Here's how the part is built. I have some questions about the finished solid (model axes, mm). Coordinates: 2 decimals unless noted, no trailing zeros. Order: outer loops, then holes, each group sorted by start corner. A loop starts at its lowest first (then second) coordinate and runs counter-clockwise, first axis right, second up. Notation, with made-up numbers: (53, -33.5) - (95, -33.5) arc R34 cw to (95, -3.5) - close; hole circle Ø4 at (4.5, -2). An arc over 180 degrees is marked (long way). Answer as CSV lines item,"result". Start each with the question number.
Q1. Suppose I cut it at B-B (x = -20). Please give me the cut outline in (y, z).
Q2. Thinking about a two-plate mould opening in Y: for faces 1 (the face through (-0.327, 17.894, 0.11)), 2 (the face through (0.355, 10, 0)), 3 (the face through (-1, 1.976, 0)), which applies, released by +Y, released by -Y, zero draft, split by the parting line, or undercut?
Q3. I need wall thicknesses on line 1 (X direction, y = 14.25, z = 3); line 2 (X direction, y = 17, z = -0.25); line 3 (Y direction, x = -7.25, z = 5). Which ranges of each line are inside material? Lowest first, please.
Q4. For pin 1 Ø12 at (x, y) = (-11, 6) entering from +Z; pin 2 Ø6 at (y, z) = (0, -1.5) entering from -X; pin 3 Ø0.9 at (x, z) = (-0.5, 1) entering from -Y, each with a flat end and sliding along its axis, tell me the tip position at first contact or that it passes through.
Q5. Suppose I cut it at A-A (y = 10). Please give me the cut outline in (x, z).
from build123d import *

# Parameters (mm, degrees)
SALIENTE_EXTRUIR1_DEPTH             = 7.21
SALIENTE_EXTRUIR2_DEPTH             = 7.21
SALIENTE_EXTRUIR2_DEPTH_BACK        = 7.21
CORTAR_EXTRUIR2_DEPTH               = 28.232395202
CORTAR_EXTRUIR2_DEPTH_BACK          = 28.232395202
SALIENTE_EXTRUIR3_REACH             = 29.232
SALIENTE_EXTRUIR3_DIRECTION_2_REACH = 29.232


with BuildPart() as part:
    # Croquis1 → Saliente-Extruir1 (new, symmetric)
    with BuildSketch(Plane.XY):
        with BuildLine():
            add(Edge.make_bspline(
                [(-18.945192114, 7.540918896), (-10.215008384, -3.697644103), (-2.846604825, -5.059081104)],
                knots=[0.497667241, 0.497667241, 0.497667241, 0.49955428, 0.49955428, 0.49955428], degree=2, weights=[1, 1, 1]))
            add(Edge.make_bspline(
                [(-2.846604825, -5.059081104), (-0.742366882, -3.9352066), (0.355125, -2.723253227)],
                knots=[0.498812075, 0.498812075, 0.498812075, 0.499412845, 0.499412845, 0.499412845], degree=2, weights=[1, 1, 1]))
            Line((0.355125, -2.723253227), (0.355125, -2.284841781))
            Line((0.355125, -2.284841781), (-1.394875, -2.223730435))
            add(Edge.make_bspline(
                [(-1.394875, -2.223730435), (-0.90753067, -0.123730435), (-1.394875, 1.976269565)],
                knots=[0, 0, 0, 1, 1, 1], degree=2, weights=[1, 3.231801219, 1]))
            Line((-1.394875, 1.976269565), (0.355125, 2.284841781))
            Line((0.355125, 2.284841781), (0.355125, 3.001549529))
            add(Edge.make_bspline(
                [(0.355125, 3.001549529), (-1.44872627, 6.058427314), (-6.994875026, 10.477389992)],
                knots=[0.500820705, 0.500820705, 0.500820705, 0.502013312, 0.502013312, 0.502013312], degree=2, weights=[1, 1, 1]))
            Line((-6.994875026, 10.477389992), (-8.981845695, 12.608155172))
            Line((-8.981845695, 12.608155172), (-23.035921146, 11.871612288))
            Line((-23.035921146, 11.871612288), (-23.035921146, 11.54013782))
            ThreePointArc((-23.035921146, 11.54013782), (-20.949684518, 9.582335705), (-18.945192114, 7.540918896))
        make_face()
    extrude(amount=SALIENTE_EXTRUIR1_DEPTH, both=True)

    # Croquis4 → Saliente-Extruir2 (add, two sides: drawn at the far end of the back side and taken through both)
    with BuildSketch(Plane.XY.offset(-SALIENTE_EXTRUIR2_DEPTH_BACK)):
        Polygon((-1.394875, 1.976269565), (0.355125, 2.284841781), (0.355125, 1.976269565), align=None)
    extrude(amount=SALIENTE_EXTRUIR2_DEPTH + SALIENTE_EXTRUIR2_DEPTH_BACK)

    # Croquis6 → Cortar-Extruir2 (cut, two sides: drawn at the far end of the back side and taken through both)
    with BuildSketch(Plane(origin=(0, 0, 0), x_dir=(0, 0, -1), z_dir=(1, 0, 0)).offset(-CORTAR_EXTRUIR2_DEPTH_BACK)):
        Polygon((7.21, 12.608155172), (7.21, -5.059081104), (5.21, -5.059081104), align=None)
        Polygon((-7.21, 12.608155172), (-7.21, -5.059081104), (-5.21, -5.059081104), align=None)
    extrude(amount=CORTAR_EXTRUIR2_DEPTH + CORTAR_EXTRUIR2_DEPTH_BACK, mode=Mode.SUBTRACT)

    # Saliente-Extruir3: up to this plane
    saliente_extruir3_end = Plane(origin=(-23.035921146, 12.608155172, 7.21), z_dir=(0, 0.1124854344122626, -0.9936533736897816))
    # Croquis8 → Saliente-Extruir3 (add, up to the surface)
    with BuildSketch(Plane.XY, mode=Mode.PRIVATE) as saliente_extruir3_sk1:
        with BuildLine():
            Line((0.355125, 3.001549529), (0.355125, 17.773466106))
            Line((0.355125, 17.773466106), (-1.028564504, 18.017447899))
            Line((-1.028564504, 18.017447899), (-2.428253067, 18.139904781))
            Line((-2.428253067, 18.139904781), (-3.764520897, 17.705725043))
            Line((-3.764520897, 17.705725043), (-5.005093297, 17.046100998))
            Line((-5.005093297, 17.046100998), (-6.1122761, 16.181074987))
            Line((-6.1122761, 16.181074987), (-7.052428119, 15.136930389))
            Line((-7.052428119, 15.136930389), (-7.796983309, 13.945393009))
            Line((-7.796983309, 13.945393009), (-8.323318739, 12.642667108))
            Line((-8.323318739, 12.642667108), (-9.726428332, 12.56913325))
            add(Edge.make_bspline(
                [(-9.726428332, 12.56913325), (-1.861127424, 6.757298639), (0.355125, 3.001549529)],
                knots=[0.500548048, 0.500548048, 0.500548048, 0.502013312, 0.502013312, 0.502013312], degree=2, weights=[1, 1, 1]))
        make_face()
    saliente_extruir3_tool1 = split(extrude(saliente_extruir3_sk1.sketch, amount=SALIENTE_EXTRUIR3_REACH, mode=Mode.PRIVATE), bisect_by=saliente_extruir3_end, keep=Keep.BOTH, mode=Mode.PRIVATE)
    add(saliente_extruir3_tool1.solids().sort_by_distance((-3.047394, 12.114755, 0))[0])

    # Saliente-Extruir3 direction 2: up to this plane
    saliente_extruir3_direction_2_end = Plane(origin=(-23.035921146, 12.608155172, -7.21), z_dir=(0, 0.1124854344122626, 0.9936533736897816))
    # Croquis8 → Saliente-Extruir3 direction 2 (add, up to the surface)
    with BuildSketch(Plane.XY, mode=Mode.PRIVATE) as saliente_extruir3_direction_2_sk1:
        with BuildLine():
            Line((0.355125, 3.001549529), (0.355125, 17.773466106))
            Line((0.355125, 17.773466106), (-1.028564504, 18.017447899))
            Line((-1.028564504, 18.017447899), (-2.428253067, 18.139904781))
            Line((-2.428253067, 18.139904781), (-3.764520897, 17.705725043))
            Line((-3.764520897, 17.705725043), (-5.005093297, 17.046100998))
            Line((-5.005093297, 17.046100998), (-6.1122761, 16.181074987))
            Line((-6.1122761, 16.181074987), (-7.052428119, 15.136930389))
            Line((-7.052428119, 15.136930389), (-7.796983309, 13.945393009))
            Line((-7.796983309, 13.945393009), (-8.323318739, 12.642667108))
            Line((-8.323318739, 12.642667108), (-9.726428332, 12.56913325))
            add(Edge.make_bspline(
                [(-9.726428332, 12.56913325), (-1.861127424, 6.757298639), (0.355125, 3.001549529)],
                knots=[0.500548048, 0.500548048, 0.500548048, 0.502013312, 0.502013312, 0.502013312], degree=2, weights=[1, 1, 1]))
        make_face()
    saliente_extruir3_direction_2_tool1 = split(extrude(saliente_extruir3_direction_2_sk1.sketch, amount=-SALIENTE_EXTRUIR3_DIRECTION_2_REACH, mode=Mode.PRIVATE), bisect_by=saliente_extruir3_direction_2_end, keep=Keep.BOTH, mode=Mode.PRIVATE)
    add(saliente_extruir3_direction_2_tool1.solids().sort_by_distance((-3.047394, 12.114755, 0))[0])


solid = part.part
Here are the results:
1,outline,"(8.64, -6.76) - (12.03, -7.14) - (12.03, 7.14) - (8.64, 6.76) - close"
2,face 1,"released by +Y"
2,face 2,"zero draft"
2,face 3,"undercut"
3,line 1,"x = -7.61 to 0.36"
3,line 2,"x = -5.06 to 0.36"
3,line 3,"y = -3.43 to 14.82"
4,pin 1,"stops at z = 7.14"
4,pin 2,"stops at x = -15.1"
4,pin 3,"stops at y = -3.88"
5,outline,"(-21.38, -6.91) - (0.36, -6.91) - (0.36, 6.91) - (-21.38, 6.91) - close"
